For this review, take the finished solid that the model builds, in its own axes (mm). A direction names the side the tool comes from. Round coordinates to 2 decimals unless told otherwise and drop trailing zeros. Order: outer loops, then holes, each group sorted by start corner. A loop starts at its lowest first (then second) coordinate and runs counter-clockwise, first axis right, second up.
```python
from build123d import *

# Parameters (mm, degrees)
SKETCH1_R           = 25.4
BOSS_EXTRUDE1_DEPTH = 6
CUT_EXTRUDE2_DEPTH  = 5
CUT_EXTRUDE3_DEPTH  = 2


with BuildPart() as part:
    # Sketch1 → Boss-Extrude1 (new body)
    with BuildSketch(Plane.XY):
        Circle(SKETCH1_R)
    extrude(amount=BOSS_EXTRUDE1_DEPTH)

    # Sketch2 → Cut-Extrude2 (cut)
    with BuildSketch(Plane.XY.offset(6)):
        with BuildLine():
            Line((-11, -13), (11, -13))
            ThreePointArc((11, -13), (12.414213562, -12.414213562), (13, -11))
            Line((13, -11), (13, 11))
            ThreePointArc((13, 11), (12.414213562, 12.414213562), (11, 13))
            Line((11, 13), (10.007987241, 13))
            ThreePointArc((10.007987241, 13), (9.446903633, 12.827759135), (9.079103078, 12.37037037))
            ThreePointArc((9.079103078, 12.37037037), (7.5, 11.3), (5.920896922, 12.37037037))
            ThreePointArc((5.920896922, 12.37037037), (5.553096367, 12.827759135), (4.992012759, 13))
            Line((4.992012759, 13), (-4.992012759, 13))
            ThreePointArc((-4.992012759, 13), (-5.553096367, 12.827759135), (-5.920896922, 12.37037037))
            ThreePointArc((-5.920896922, 12.37037037), (-7.5, 11.3), (-9.079103078, 12.37037037))
            ThreePointArc((-9.079103078, 12.37037037), (-9.446903633, 12.827759135), (-10.007987241, 13))
            Line((-10.007987241, 13), (-11, 13))
            ThreePointArc((-11, 13), (-12.414213562, 12.414213562), (-13, 11))
            Line((-13, 11), (-13, -11))
            ThreePointArc((-13, -11), (-12.414213562, -12.414213562), (-11, -13))
        make_face()
    extrude(amount=-CUT_EXTRUDE2_DEPTH, mode=Mode.SUBTRACT)

    # Sketch3 → Cut-Extrude3 (cut, through all)
    with BuildSketch(Plane.XY.offset(1)):
        with BuildLine():
            Line((-10.9, -8.9), (-10.9, 9.1))
            ThreePointArc((-10.9, 9.1), (-10.314213562, 10.514213562), (-8.9, 11.1))
            Line((-8.9, 11.1), (9.1, 11.1))
            ThreePointArc((9.1, 11.1), (10.514213562, 10.514213562), (11.1, 9.1))
            Line((11.1, 9.1), (11.1, -8.9))
            ThreePointArc((11.1, -8.9), (10.514213562, -10.314213562), (9.1, -10.9))
            Line((9.1, -10.9), (2.85, -10.9))
            ThreePointArc((2.85, -10.9), (2.142893219, -10.607106781), (1.85, -9.9))
            Line((1.85, -9.9), (1.85, -9.8))
            Line((1.85, -9.8), (-1.65, -9.8))
            Line((-1.65, -9.8), (-1.65, -9.9))
            ThreePointArc((-1.65, -9.9), (-1.942893219, -10.607106781), (-2.65, -10.9))
            Line((-2.65, -10.9), (-8.9, -10.9))
            ThreePointArc((-8.9, -10.9), (-10.314213562, -10.314213562), (-10.9, -8.9))
        make_face()
    extrude(amount=-CUT_EXTRUDE3_DEPTH, mode=Mode.SUBTRACT)


solid = part.part
```
Q1. Tool access review of faces 1 (the face through (10.5, 10.53, 0.51)), 2 (the face through (7.5, 11.3, 3.5)), 3 (the face through (0, -17, 6)): name each direction out of +Z, -Z, +X, -X, +Y, -Y from which nothing blocks a thin tool from reaching the whole face with its end or side.
Q2. Wall thickness on line 1 (X direction, y = -10, z = 0.4); line 2 (Z direction, x = 12.5, y = -3); line 3 (Y direction, x = 6, z = 2.6): over which ranges is each line inside the solid? List them lowest first.
Q3. Mouldability with a two-part tool opening along Y and no side actions: class faces 4 (the face through (0, -11, 0)), 5 (the face through (-5.506, -24.796, 2.958)), 6 (the face through (-13, 0, 4)) as +Y half, -Y half, draft (parallel to the pull), parting line (faces both ways), or undercut.
Q4. Take a section at A-A, the plane z = 1.65. State the section outline as (x, y) points.
Q5. Clearance check with flat-ended pins moving along their axes: pin 1 (1 mm diameter, centred on y = -5, z = 1.5, fed in from -X); pin 2 (1.1 mm diameter, centred on x = 10.5, z = 3, fed in from -Y); pin 3 (0.8 mm diameter, centred on x = -4, z = 0.5, fed in from -Y); pin 4 (2 mm diameter, centred on x = -11.5, y = -11, fed in from -Z). State where each tip first meets the part, or that it passes through.
Q6. Take a section at C-C, the plane y = 0. State the section outline as (x, z) points.
Q7. Take a section at B-B, the plane x = 0. State the section outline as (y, z) points.
Q8. Take a section at D-D, the plane x = 16.5. State the section outline as (y, z) points, plus the area to 3 significant figures.
Working result:
1. face 1: +Z, -Z
1. face 2: +Z
1. face 3: +Z, +X, -X, +Y, -Y
2. line 1: x = -23.35 to -10.57, -1.66 to 1.86, 10.77 to 23.35
2. line 2: z = 0 to 1
2. line 3: y = -24.68 to -13, 12.2 to 24.68
3. face 4: draft
3. face 5: parting line
3. face 6: undercut
4. outline: circle Ø50.8 at (0, 0); hole (-13, -11) arc R2 ccw to (-11, -13) - (11, -13) arc R2 ccw to (13, -11) - (13, 11) arc R2 ccw to (11, 13) - (10.01, 13) arc R1 ccw to (9.08, 12.37) arc R1.7 cw to (5.92, 12.37) arc R1 ccw to (4.99, 13) - (-4.99, 13) arc R1 ccw to (-5.92, 12.37) arc R1.7 cw to (-9.08, 12.37) arc R1 ccw to (-10.01, 13) - (-11, 13) arc R2 ccw to (-13, 11) - close
5. pin 1: stops at x = -25
5. pin 2: stops at y = -23.37
5. pin 3: stops at y = -25.14
5. pin 4: stops at z = 0
6. outline: (-25.4, 0) - (-10.9, 0) - (-10.9, 1) - (-13, 1) - (-13, 6) - (-25.4, 6) - close; (11.1, 0) - (25.4, 0) - (25.4, 6) - (13, 6) - (13, 1) - (11.1, 1) - close
7. outline: (-25.4, 0) - (-9.8, 0) - (-9.8, 1) - (-13, 1) - (-13, 6) - (-25.4, 6) - close; (11.1, 0) - (25.4, 0) - (25.4, 6) - (13, 6) - (13, 1) - (11.1, 1) - close
8. outline: (-19.31, 0) - (19.31, 0) - (19.31, 6) - (-19.31, 6) - close
8. area: 232 mm2
